Input: part model. Units: mm. Frame: model coordinates. Round coordinates to 2 decimals unless told otherwise and drop trailing zeros. Write each loop counter-clockwise with the first axis right and the second up, starting at its lowest first coordinate (ties: lowest second). Pieces come first, ordered by that corner, then holes. Notation, with made-up numbers: (-24.75, -28.5) - (25.25, -28.5) arc R25 ccw to (25.25, -6.5) - close; hole circle Ø5 at (82.5, -13.75). An arc over 180 degrees is marked (long way). Use one line per item in the form item = value.
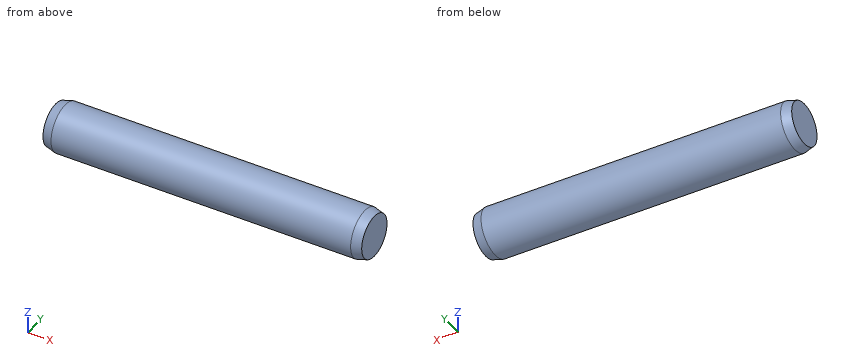
```python
from build123d import *

# Parameters (mm, degrees)
SKETCH2_R           = 3
EXTRUDE1_DEPTH      = 18.8
EXTRUDE1_DEPTH_BACK = 18.8
SKETCH3_R           = 3
EXTRUDE2_DEPTH      = 1.2
EXTRUDE2_TAPER      = 15
SKETCH4_R           = 3
EXTRUDE3_DEPTH      = 1.2
EXTRUDE3_TAPER      = 15


with BuildPart() as part:
    # Sketch2 → Extrude1 (new body, two sides)
    with BuildSketch(Plane(origin=(0, 0, 0), x_dir=(0, 0, -1), z_dir=(1, 0, 0))) as extrude1_sk:
        Circle(SKETCH2_R)
    extrude(amount=EXTRUDE1_DEPTH)
    extrude(extrude1_sk.sketch, amount=-EXTRUDE1_DEPTH_BACK)

    # Sketch3 → Extrude2 (add)
    with BuildSketch(Plane(origin=(18.8, 0, 0), x_dir=(0, 0, -1), z_dir=(1, 0, 0))):
        Circle(SKETCH3_R)
    extrude(amount=EXTRUDE2_DEPTH, taper=EXTRUDE2_TAPER)

    # Sketch4 → Extrude3 (add)
    with BuildSketch(Plane.ZY.offset(18.8)):
        Circle(SKETCH4_R)
    extrude(amount=EXTRUDE3_DEPTH, taper=EXTRUDE3_TAPER)


solid = part.part
```
(1) Cut plane A-A on x = -4. Output: boundary loops of the cut face in (y, z), then the cut area to 3 significant figures.
Derived:
outline = circle Ø6 at (0, 0)
area = 28.3 mm^2
(2) First-contact query: pin 1 Ø3 at (x, y) = (15, -0.5) entering from -Z. Flat tip, straight axial feed; report the tip coordinate or a pass-through.
Derived:
pin_1 = -3
(3) Material intervals for L1, parallel to Z at x = 5, y = -2.5; L2, parallel to Z at x = -12.5, y = -0.5; L3, parallel to Y at x = -5.5, z = -0.25, sorted ascending.
Derived:
L1 = -1.66 to 1.66
L2 = -2.96 to 2.96
L3 = -2.99 to 2.99
